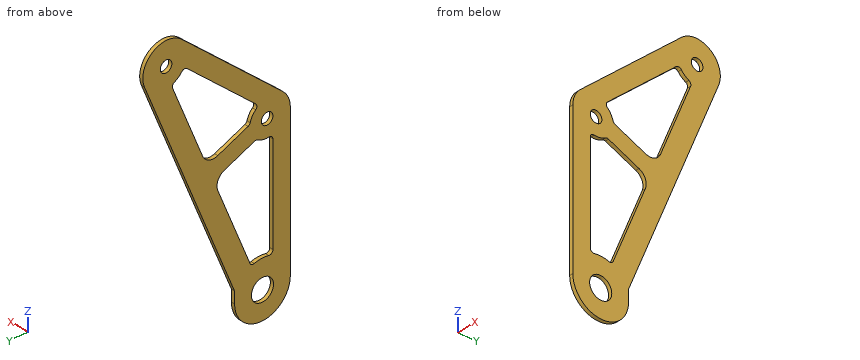
```python
from build123d import *

# Parameters (mm, degrees)
BOSS_EXTRUDE1_DEPTH         = 3
F_3_4_0_75_DIAMETER_HOLE1_D = 19.05
F_10_0_10_DIAMETER_HOLE1_D  = 10
F_10_0_10_DIAMETER_HOLE2_D  = 10
CUT_EXTRUDE1_REACH          = 210.238


with BuildPart() as part:
    # Sketch1 → Boss-Extrude1 (new body)
    with BuildSketch(Plane(origin=(0, 0, 0), x_dir=(0, 0, -1), z_dir=(1, 0, 0))):
        with BuildLine():
            Line((-65, 0), (65, 0))
            ThreePointArc((65, 0), (89, 24), (65, 48))
            Line((65, 48), (55, 48))
            Line((55, 48), (-137.527302422, 125.551517213))
            ThreePointArc((-137.527302422, 125.551517213), (-161.448822218, 118.377005214), (-159.721992414, 93.462535711))
            Line((-159.721992414, 93.462535711), (-79.721992414, 6.462535711))
            ThreePointArc((-79.721992414, 6.462535711), (-73.038989807, 1.686763178), (-65, 0))
        make_face()
    extrude(amount=BOSS_EXTRUDE1_DEPTH)

    # 3/4 (0.75) Diameter Hole1 (through all)
    with Locations(Plane(origin=(3, 0, 0), x_dir=(0, 0, -1), z_dir=(1, 0, 0))):
        with Locations((65, 24)):
            Hole(F_3_4_0_75_DIAMETER_HOLE1_D / 2)

    # Ø10.0 (10) Diameter Hole1 (through all)
    with Locations(Plane(origin=(3, 0, 0), x_dir=(0, 0, -1), z_dir=(1, 0, 0))):
        with Locations((-145, 107)):
            Hole(F_10_0_10_DIAMETER_HOLE1_D / 2)

    # Ø10.0 (10) Diameter Hole2 (through all)
    with Locations(Plane(origin=(3, 0, 0), x_dir=(0, 0, -1), z_dir=(1, 0, 0))):
        with Locations((-65, 20)):
            Hole(F_10_0_10_DIAMETER_HOLE2_D / 2)

    # Sketch8 → Cut-Extrude1 (cut, up to next)
    with BuildSketch(Plane(origin=(3, 0, 0), x_dir=(0, 0, -1), z_dir=(1, 0, 0)), mode=Mode.PRIVATE) as cut_extrude1_sk1:
        with BuildLine():
            Line((38.136909616, 15), (-47.11145618, 15))
            ThreePointArc((-47.11145618, 15), (-49.347524158, 16), (-50.09288015, 18.333333333))
            ThreePointArc((-50.09288015, 18.333333333), (-50.384311526, 23.373670173), (-52.331533313, 28.031808751))
            ThreePointArc((-52.331533313, 28.031808751), (-52.785410617, 29.365367154), (-52.580567558, 30.759075138))
            Line((-52.580567558, 30.759075138), (-42.048503485, 56.905692997))
            ThreePointArc((-42.048503485, 56.905692997), (-36.689699124, 62.370293585), (-29.036396089, 62.445102815))
            Line((-29.036396089, 62.445102815), (39.768193948, 34.730070809))
            ThreePointArc((39.768193948, 34.730070809), (41.351904066, 33.245441463), (41.519519359, 31.08114778))
            ThreePointArc((41.519519359, 31.08114778), (40.491403893, 24.896851079), (41.064766878, 18.653950954))
            ThreePointArc((41.064766878, 18.653950954), (40.478047465, 16.124080607), (38.136909616, 15))
        make_face()
    cut_extrude1_tool1 = extrude(cut_extrude1_sk1.sketch, amount=-CUT_EXTRUDE1_REACH, mode=Mode.PRIVATE) & part.part
    # Sketch8 → Cut-Extrude1 (cut, up to next)
    with BuildSketch(Plane(origin=(3, 0, 0), x_dir=(0, 0, -1), z_dir=(1, 0, 0)), mode=Mode.PRIVATE) as cut_extrude1_sk2:
        with BuildLine():
            Line((-135.210891206, 88.967436427), (-80.78877426, 29.783384249))
            ThreePointArc((-80.78877426, 29.783384249), (-78.53914012, 28.814288673), (-76.317062832, 29.845003243))
            ThreePointArc((-76.317062832, 29.845003243), (-72.806710034, 32.808406554), (-68.564110875, 34.570419132))
            ThreePointArc((-68.564110875, 34.570419132), (-67.312603666, 35.217035191), (-66.494205468, 36.363598321))
            Line((-66.494205468, 36.363598321), (-55.962141395, 62.51021618))
            ThreePointArc((-55.962141395, 62.51021618), (-56.036950624, 70.163519215), (-61.501551212, 75.522323576))
            Line((-61.501551212, 75.522323576), (-125.724416937, 101.391800861))
            ThreePointArc((-125.724416937, 101.391800861), (-127.951011637, 101.397881175), (-129.568523338, 99.867712287))
            ThreePointArc((-129.568523338, 99.867712287), (-131.78341646, 96.307857113), (-134.802203492, 93.39834766))
            ThreePointArc((-134.802203492, 93.39834766), (-135.989912088, 91.27359327), (-135.210891206, 88.967436427))
        make_face()
    cut_extrude1_tool2 = extrude(cut_extrude1_sk2.sketch, amount=-CUT_EXTRUDE1_REACH, mode=Mode.PRIVATE) & part.part
    add(cut_extrude1_tool1.solids().sort_by_distance((3, 33.678975, 9.935065))[0], mode=Mode.SUBTRACT)
    add(cut_extrude1_tool2.solids().sort_by_distance((3, 67.393587, 91.526905))[0], mode=Mode.SUBTRACT)


solid = part.part
```
For this review, take the finished solid that the model builds, in its own axes (mm). Round coordinates to 2 decimals unless told otherwise and drop trailing zeros. Write each loop counter-clockwise with the first axis right and the second up, starting at its lowest first coordinate (ties: lowest second). Pieces come first, ordered by that corner, then holes. Notation, with made-up numbers: (85, 81.5) - (131, 81.5) arc R10 cw to (131, 98.5) - close; hole circle Ø11 at (43.5, 80). An arc over 180 degrees is marked (long way). Answer as CSV lines item,"result". Start each with the question number.
(1) For pin 1 (13 mm diameter, centred on y = 20, z = 65, fed in from -X); pin 2 (1.5 mm diameter, centred on x = 2, z = -60.5, fed in from +Y), all flat-tipped, find the tip position at first contact; note any pin that passes through.
(2) Add section C-C, the plane x = 2.3. State how many separate pieces and enclosed holes the cut face has, plus the area to 3 significant figures.
(3) Add section A-A, the plane z = 145. State the section outline as (x, y) points, plus the area to 3 significant figures.
(4) Add section D-D, the plane y = 117.5. State the section outline as (x, z) points, plus the area to 3 significant figures.
(5) For line 1 (Z direction, x = 1.85, y = 54.5); line 2 (Y direction, x = 2.4, z = -65) (3 decimals); line 3 (Y direction, x = 1.8, z = 65), list the stretches that pass through material, from the lowest coordinate up.
(6) Add section B-B, the plane y = 81. State the section outline as (x, z) points.
From the geometry:
1,pin 1,"stops at x = 0"
1,pin 2,"stops at y = 48"
2,separate pieces,"1"
2,enclosed holes,"5"
2,area,"10,500 mm²"
3,outline,"(0, 77.45) - (3, 77.45) - (3, 102) - (0, 102) - close; (0, 112) - (3, 112) - (3, 127) - (0, 127) - close"
3,area,"119 mm²"
4,outline,"(0, 117.54) - (3, 117.54) - (3, 162.02) - (0, 162.02) - close"
4,area,"133 mm²"
5,line 1,"z = -38.86 to 9.31, 43.02 to 59.19, 103.52 to 123.89"
5,line 2,"y = 0 to 14.475, 33.525 to 48"
5,line 3,"y = 0 to 15, 25 to 40.07, 76.93 to 96.34"
6,outline,"(0, 26.92) - (3, 26.92) - (3, 75.1) - (0, 75.1) - close; (0, 127.88) - (3, 127.88) - (3, 148.26) - (0, 148.26) - close"
